Could you check a few things on this model? Use its own coordinates, in mm. A direction names the side the tool comes from. Give positions to 0.01 mm unless a question says otherwise; leave off trailing zeros. Loops run counter-clockwise (first coordinate to the right, second up) from the corner with the lowest first, then second, coordinate; pieces in that order, holes last. Notation, with made-up numbers: M 63.5,7 L 76.5,7 A12 ccw 76.5,24 Z; hole C -33.75,25.5 d5. An arc over 180 degrees is marked long. Answer in a Markdown table with one row per item. Add a question column.
1. Thinking about a two-plate mould opening in X: for faces 1 (the cylindrical face through (58.57, 30.6, -2.46)), 2 (the flat face through (86.7, 18.7, -2)), 3 (the flat face through (39, 24, -5)), which applies, released by +X, released by -X, zero draft, split by the parting line, or undercut?
2. If we section it at B-B on y = 20: List the corners of the cut face in (x, z) for me, then the cut area to 3 significant figures.
3. I need wall thicknesses on line 1 along Y through (x, z) = (88, -4.35); line 2 along X through (y, z) = (20, -0.75); line 3 along Y through (x, z) = (57, -1.9). Which ranges of each line are inside material? Lowest first, please. Write a range as from..to.
4. If we section it at C-C on z = -1.1: List the corners of the cut face in (x, y) for me.
5. If we section it at A-A on x = 88: List the corners of the cut face in (y, z) for me, then the cut area to 3 significant figures.
6. I'm going to push flat-ended pins straight in: pin 1 Ø2 at (x, z) = (50, -1) entering from +Y; pin 2 Ø2.5 at (x, z) = (77.5, -3) entering from -Y; pin 3 Ø2.5 at (y, z) = (5, -3.5) entering from +X. Where does each tip first touch, or does it pass through?
7. If we section it at D-D on x = 14: List the corners of the cut face in (y, z) for me.
8. Which directions (+Z, -Z, +X, -X, +Y, -Y) give clear straight access to the entire face, cutting with the end or side of a thin tool? Please do faces 4 (the cylindrical face through (85, 20, -4)), 5 (the flat face through (78, 10, -3)), 6 (the cylindrical face through (11.015, 43.244, -2.535)).
Autodesk Inventor part; units mm, degrees
ref_plane "YZ Plane" through (0, 0, 0) normal (1, 0, 0) x (0, 1, 0)
ref_plane "XZ Plane" through (0, 0, 0) normal (0, 1, 0) x (-1, 0, 0)
ref_plane "XY Plane" through (0, 0, 0) normal (0, 0, 1) x (1, 0, 0)
sketch "スケッチ1" plane through (0, 0, 0) normal (0, 0, 1) x (1, 0, 0)
  line L0 (0, 0) -> (98, 0)
  line L1 (98, 0) -> (98, 60)
  line L2 (98, 60) -> (0, 60)
  line L3 (0, 60) -> (0, 0)
  line L4 (98, 0) -> (29, 0)
  line L5 (29, 0) -> (29, 40)
  line L6 (29, 40) -> (98, 40)
  line L7 (98, 40) -> (98, 0)
  line L8 (29, 30) -> (98, 30)
  line L9 (98, 30) -> (98, 10)
  line L10 (98, 10) -> (29, 10)
  line L11 (29, 10) -> (29, 30)
  line L12 (98, 20) -> (0, 20)
  line L13 (29, 20) -> (5.906, 60)
  circle A0 centre (29, 20) radius 8
  circle A1 centre (14, 45.9808) radius 4.05
  line L14 (58, 40) -> (58, 0)
  line L15 (16.8756, 13) -> (-6.2184, 53)
  line L16 (41.1244, 27) -> (18.0303, 67)
  circle A2 centre (14, 45.9808) radius 14
  line L17 (16.8756, 13) -> (25.3526, -1.6825)
  point P0 (58, 30)
  point P1 (33.6188, 40)
  point P2 (22.0718, 60)
  point P3 (0, 45.9808)
  point P4 (1.8756, 38.9808)
  point P5 (24.3812, 0)
  point P6 (58, 0)
  point P7 (58, 10)
  dimension "d0" = 98
  dimension "d1" = 60
  dimension "d2" = 40
  dimension "d3" = 20
  dimension "d4" = 10
  dimension "d5" = 69
  dimension "d6" = 30
  dimension "d7" = 16
  dimension "d8" = 30
  dimension "d9" = 8.1
  dimension "d10" = 40
  dimension "d11" = 28
extrude "押し出し1" add sketch "スケッチ1" along normal blind 5 contours L5 L10 L14 L0 | L0 L17 L15 L12 A0 L5 | L5 A0 L12 L14 L10 | L14 L12 L1 L10 | L14 L8 L1 L12 | L12 A0 L5 L8 L14 | L15 A2 L13 A0 L12 | L8 L16 L6 L14 | A2 L13 A1 | A0 L13 A2 L16 L6 L5 | L8 L5 L6 L16 | L3 L2 L13 A2 | L13 A1 A2 | L13 L2 L16 A2
sketch "スケッチ2" plane through (0, 0, 5) normal (0, 0, 1) x (1, 0, 0)
  line L0 (98, 10) -> (98, 30)
  line L1 (98, 20) -> (47.1161, 20)
  point P0 (0, 0)
  point P1 (88, 20)
  point P2 (58, 20)
  dimension "d14" = 10
  dimension "d15" = 30
hole "穴1" at (88, 20, 5) at (58, 20, 5) direction (0, 0, -1) diameter 3.2 depth 10
fillet "フィレット1" radius 2 6 edges at (58, 40, 2.5) (58, 30, 2.5) (98, 30, 2.5) (98, 10, 2.5) (58, 0, 2.5) (58, 10, 2.5)
fillet "フィレット2" radius 10 4 edges at (24.3812, 0, 2.5) (0, 60, 2.5) (22.0718, 60, 2.5) (33.6188, 40, 2.5)
sketch "スケッチ4" plane through (0, 0, 5) normal (0, 0, 1) x (1, 0, 0)
  circle A0 centre (58, 20) radius 1.6
  circle A1 centre (58, 20) radius 3
  circle A2 centre (88, 20) radius 1.6
  circle A3 centre (88, 20) radius 3
  point P0 (0, 0)
  dimension "d34" = 6
  dimension "d35" = 6
extrude "押し出し2" cut sketch "スケッチ4" against normal blind 3 contours A0 | A1 | A2 | A3
mirror "ミラー1" about plane through (0, 0, 0) normal (0, 0, 1)
sketch "スケッチ5" plane through (0, 0, 5) normal (0, 0, 1) x (1, 0, 0)
  line L0 (-47.2923, 84.9681) -> (163.8235, 84.9681)
  line L1 (163.8235, 84.9681) -> (163.8235, -15.7821)
  line L2 (163.8235, -15.7821) -> (-47.2923, -15.7821)
  line L3 (-47.2923, -15.7821) -> (-47.2923, 84.9681)
  point P0 (0, 0)
extrude "押し出し3" cut sketch "スケッチ5" against normal blind 5
equation "\"d35\" = d34"
properties part number "RP_Calf-Link-cover-Outside-Left"
Results:
| question | item | result |
|---|---|---|
| 1 | face 1 | released by +X |
| 1 | face 2 | undercut |
| 1 | face 3 | zero draft |
| 2 | outline | M 12.83,-5 L 21,-5 L 21,0 L 12.83,0 Z; M 37,-5 L 55,-5 L 55,-2 L 56.4,-2 L 56.4,0 L 37,0 Z; M 59.6,-2 L 61,-2 L 61,-5 L 85,-5 L 85,-2 L 86.4,-2 L 86.4,0 L 59.6,0 Z; M 89.6,-2 L 91,-2 L 91,-5 L 98,-5 L 98,0 L 89.6,0 Z |
| 2 | area | 297 mm2 |
| 3 | line 1 | 10..17, 23..30 |
| 3 | line 2 | 12.83..21, 37..56.4, 59.6..86.4, 89.6..98 |
| 3 | line 3 | 0.27..18.75, 21.25..39.73 |
| 4 | outline | M 0,45.98 A14 ccw 1.88,38.98 L 16.88,13 L 21.49,5 A10 ccw 30.15,0 L 56,0 A2 ccw 58,2 L 58,8 A2 cw 60,10 L 96,10 A2 ccw 98,12 L 98,28 A2 ccw 96,30 L 60,30 A2 cw 58,32 L 58,38 A2 ccw 56,40 L 39.39,40 A10 cw 30.73,45 L 24.96,55 A10 ccw 16.3,60 L 10,60 A10 ccw 0,50 Z; hole C 14,45.98 d8.1; hole C 29,20 d16; hole C 58,20 d3.2; hole C 88,20 d3.2 |
| 5 | outline | M 10,-5 L 17,-5 L 17,-2 L 18.4,-2 L 18.4,0 L 10,0 Z; M 21.6,-2 L 23,-2 L 23,-5 L 30,-5 L 30,0 L 21.6,0 Z |
| 5 | area | 75.6 mm2 |
| 6 | pin 1 | y = 40 |
| 6 | pin 2 | y = 10 |
| 6 | pin 3 | x = 58 |
| 7 | outline | M 17.98,-5 L 41.93,-5 L 41.93,0 L 17.98,0 Z; M 50.03,-5 L 60,-5 L 60,0 L 50.03,0 Z |
| 8 | face 4 | -Z |
| 8 | face 5 | +Z, -Z, +X, -Y |
| 8 | face 6 | +Z, -Z |
